```python
from build123d import *

# Parameters (mm, degrees)
F0_W     = 152.4
F0_H     = 254
F1_DEPTH = 6.35
F3_DEPTH = 25.4
F6_D     = 4.4958


with BuildPart() as f1:
    # F0 (on Top) → F1 (new body)
    with BuildSketch(Plane.XY):
        Rectangle(F0_W, F0_H)
    extrude(amount=F1_DEPTH)

    # F2 (on face) → F3 (cut)
    with BuildSketch(Plane.XY.offset(6.35)):
        with BuildLine():
            Line((-58.3057, 116.5479), (-63.3857, 116.5479))
            ThreePointArc((-63.3857, 116.5479), (-65.6336, 114.3), (-63.3857, 112.0521))
            Line((-63.3857, 112.0521), (-58.3057, 112.0521))
            ThreePointArc((-58.3057, 112.0521), (-56.0578, 114.3), (-58.3057, 116.5479))
        make_face()
        with BuildLine():
            Line((63.3857, 116.5479), (58.3057, 116.5479))
            ThreePointArc((58.3057, 116.5479), (56.0578, 114.3), (58.3057, 112.0521))
            Line((58.3057, 112.0521), (63.3857, 112.0521))
            ThreePointArc((63.3857, 112.0521), (65.6336, 114.3), (63.3857, 116.5479))
        make_face()
        with BuildLine():
            Line((-58.3057, 14.9479), (-63.3857, 14.9479))
            ThreePointArc((-63.3857, 14.9479), (-65.6336, 12.7), (-63.3857, 10.4521))
            Line((-63.3857, 10.4521), (-58.3057, 10.4521))
            ThreePointArc((-58.3057, 10.4521), (-56.0578, 12.7), (-58.3057, 14.9479))
        make_face()
        with BuildLine():
            Line((63.3857, 14.9479), (58.3057, 14.9479))
            ThreePointArc((58.3057, 14.9479), (56.0578, 12.7), (58.3057, 10.4521))
            Line((58.3057, 10.4521), (63.3857, 10.4521))
            ThreePointArc((63.3857, 10.4521), (65.6336, 12.7), (63.3857, 14.9479))
        make_face()
    extrude(amount=-F3_DEPTH, mode=Mode.SUBTRACT)

    # F6 (through all)
    with Locations(Plane.XY.offset(6.35)):
        with Locations((-63.5, -19.05), (-63.5, -114.3), (63.5, -114.3), (63.5, -19.05), (-25.4, 114.3), (25.4, 114.3)):
            Hole(F6_D / 2)


solid = f1.part
```
Verification items for the finished model (mm, model axes). A direction names the side the tool comes from. Give positions to 0.01 mm unless a question says otherwise; leave off trailing zeros. Answer in a Markdown table with one row per item. Add a question column.
Item 1: Tool access check on faces 1 (the flat face through (-1, 2, 6.35)), 2 (the cylindrical face through (56.06, 114.35, 3.22)). Record the directions out of +Z, -Z, +X, -X, +Y, -Y that give a thin tool (end or side, any length) a straight path to the whole face; none if there is none.
Item 2: Scan lines: probe 1 along Y at (x, z) = (-63.5, 3) (3 decimals); probe 2 along Y at (x, z) = (25.4, 4.5). Record each from-to range of solid material in increasing order. Write a range as from..to.
Item 3: Mould release check, pull along Y, two halves, no side actions. Record for faces 3 (the flat face through (-1, -127, 3)), 4 (the flat face through (-1, 2, 0)), 5 (the cylindrical face through (65.633, 114.251, 3.219)): released by +Y, released by -Y, zero draft, split by the parting line, or undercut.
Filled sheet:
| question | item | result |
|---|---|---|
| 1 | face 1 | +Z, +X, -X, +Y, -Y |
| 1 | face 2 | +Z, -Z |
| 2 | probe 1 | y = -127..-116.548, -112.052..-21.298, -16.802..10.455, 14.945..112.055, 116.545..127 |
| 2 | probe 2 | y = -127..112.05, 116.55..127 |
| 3 | face 3 | released by -Y |
| 3 | face 4 | zero draft |
| 3 | face 5 | undercut |
